Input: part model. Units: mm. Frame: model coordinates. A direction names the side the tool comes from. Round coordinates to 2 decimals unless told otherwise and drop trailing zeros. Order: outer loops, then holes, each group sorted by start corner. A loop starts at its lowest first (then second) coordinate and runs counter-clockwise, first axis right, second up. Notation, with made-up numbers: (70.5, -33) -> (104.5, -33) arc R23 ccw to (104.5, -16) -> close; hole circle Ø3 at (57.5, -4.75). An arc over 180 degrees is marked (long way). Use a Markdown table: item, result.
from build123d import *

# Parameters (mm, degrees)
F0_W      = 1000
F0_H      = 1000
F1_DEPTH  = 300
F2_W      = 900
F2_H      = 100
F3_DEPTH  = 1000.001
F4_W      = 100
F4_H      = 900
F5_DEPTH  = 1000.001
F6_W      = 300
F6_H      = 120
F7_DEPTH  = 150
F8_W      = 300
F8_H      = 120
F9_DEPTH  = 150
F10_W     = 120
F10_H     = 300
F11_DEPTH = 150
F12_W     = 120
F12_H     = 300
F13_DEPTH = 150
F14_R     = 5
F15_R     = 5
F16_W     = 680
F16_H     = 680
F17_DEPTH = 300.001
F18_W     = 10
F18_H     = 680
F19_DEPTH = 160.001
F20_DEPTH = 840.001
F21_SCALE = 0.1


with BuildPart() as f1:
    # F0 (on Front) → F1 (new body)
    with BuildSketch(Plane.XZ):
        with Locations((450.7653813809, 448.8989327101)):
            Rectangle(F0_W, F0_H)
    extrude(amount=F1_DEPTH)

    # F2 (on face) → F3 (cut, through all)
    with BuildSketch(Plane.XY.offset(948.8989327101)):
        with Locations((450.7653813809, -250)):
            Rectangle(F2_W, F2_H)
    extrude(amount=-F3_DEPTH, mode=Mode.SUBTRACT)

    # F4 (on face) → F5 (cut, through all)
    with BuildSketch(Plane(origin=(-49.2346186191, 0, 0), x_dir=(0, -1, 0), z_dir=(-1, 0, 0))):
        with Locations((250, 448.8989327101)):
            Rectangle(F4_W, F4_H)
    extrude(amount=-F5_DEPTH, mode=Mode.SUBTRACT)

    # F6 (on face) → F7 (cut)
    with BuildSketch(Plane(origin=(0, 0, -51.1010672899), x_dir=(1, 0, 0), z_dir=(0, 0, -1))):
        with Locations((100.7653813809, 110)):
            Rectangle(F6_W, F6_H)
    extrude(amount=-F7_DEPTH, mode=Mode.SUBTRACT)

    # F8 (on face) → F9 (cut)
    with BuildSketch(Plane(origin=(0, 0, -51.1010672899), x_dir=(1, 0, 0), z_dir=(0, 0, -1))):
        with Locations((800.7653813809, 110)):
            Rectangle(F8_W, F8_H)
    extrude(amount=-F9_DEPTH, mode=Mode.SUBTRACT)

    # F10 (on face) → F11 (cut)
    with BuildSketch(Plane.YZ.offset(950.7653813809)):
        with Locations((-110, 798.8989327101)):
            Rectangle(F10_W, F10_H)
    extrude(amount=-F11_DEPTH, mode=Mode.SUBTRACT)

    # F12 (on face) → F13 (cut)
    with BuildSketch(Plane(origin=(-49.2346186191, 0, 0), x_dir=(0, -1, 0), z_dir=(-1, 0, 0))):
        with Locations((110, 798.8989327101)):
            Rectangle(F12_W, F12_H)
    extrude(amount=-F13_DEPTH, mode=Mode.SUBTRACT)

    # F14
    f14_edges = [f1.edges().sort_by_distance(p)[0] for p in [
        (950.765381, -235, -51.101067),
        (900.765381, -250, -51.101067),
        (950.765381, -250, -1.101067),
        (900.765381, -250, -1.101067),
        (-49.234619, -235, -51.101067),
        (0.765381, -250, -51.101067),
        (-49.234619, -250, -1.101067),
        (0.765381, -250, -1.101067),
        (-49.234619, -235, 948.898933),
        (0.765381, -250, 948.898933),
        (-49.234619, -250, 898.898933),
        (0.765381, -250, 898.898933),
        (950.765381, -235, 948.898933),
        (950.765381, -250, 898.898933),
        (900.765381, -250, 898.898933),
        (900.765381, -250, 948.898933),
    ]]
    fillet(f14_edges, radius=F14_R)

    # F15
    f15_edges = [f1.edges().sort_by_distance(p)[0] for p in [
        (950.765381, -25, 948.898933),
        (950.765381, -25, -51.101067),
        (-49.234619, -25, -51.101067),
        (-49.234619, -25, 948.898933),
    ]]
    fillet(f15_edges, radius=F15_R)

    # F16 (on face) → F17 (cut, through all)
    with BuildSketch(Plane(origin=(0, 0, 0), x_dir=(-1, 0, 0), z_dir=(0, 1, 0))):
        with Locations((-450.7653813809, 448.8989327101)):
            Rectangle(F16_W, F16_H)
    extrude(amount=-F17_DEPTH, mode=Mode.SUBTRACT)

    # F18 (on face) → F19 (cut, through all)
    with BuildSketch(Plane.YZ.offset(110.7653813809)):
        with Locations((-10, 445.622831583)):
            Rectangle(F18_W, F18_H)
    extrude(amount=-F19_DEPTH, mode=Mode.SUBTRACT)

    # F18 (on face) → F20 (cut, through all)
    with BuildSketch(Plane.YZ.offset(110.7653813809)):
        with Locations((-10, 445.622831583)):
            Rectangle(F18_W, F18_H)
    extrude(amount=F20_DEPTH, mode=Mode.SUBTRACT)


with BuildPart() as f1_1:
    # F21: moved
    add(f1.part.scale(F21_SCALE))


solid = f1_1.part
1) Cut plane B-B on x = 13.5. Return loops of the section in (y, z), and give its area (3 significant figures).
Results found:
| item | result |
|---|---|
| outline | (-20, -5.11) -> (-17, -5.11) -> (-17, 9.89) -> (-5, 9.89) -> (-5, -5.11) -> (0, -5.11) -> (0, 10.89) -> (-0.5, 10.89) -> (-0.5, 10.56) -> (-1.5, 10.56) -> (-1.5, 10.89) -> (-20, 10.89) -> close; (-20, 78.89) -> (0, 78.89) -> (0, 94.89) -> (-20, 94.89) -> close |
| area | 460 mm² |
2) Cut plane A-A on y = -24.25. Count the separate pieces of the cut face and the enclosed holes in it, and give its area (3 significant figures).
Results found:
| item | result |
|---|---|
| separate pieces | 4 |
| enclosed holes | 0 |
| area | 99.1 mm² |
3) Set-up query: faces 1 (the flat face through (10, -5, 2)), 2 (the flat face through (-2, -25, -0.11)), 3 (the flat face through (11.077, -12, 44)). Return all of +Z, -Z, +X, -X, +Y, -Y with unobstructed straight access to the full face (end or side cutting, diameter ignored); none if empty.
Results found:
| item | result |
|---|---|
| face 1 | -Z, -X |
| face 2 | +X, -X, -Y |
| face 3 | +Y, -Y |
4) Pull-direction query (Y, two-part tool) for faces 4 (the flat face through (-4.923, -11, 44)), 5 (the flat face through (-2, -30, -3)), 6 (the flat face through (80, -11, 9.89)), 7 (the flat face through (8, -1.5, 42)); classes: +Y half, -Y half, draft (parallel to the pull), parting line (faces both ways), or undercut.
Results found:
| item | result |
|---|---|
| face 4 | draft |
| face 5 | -Y half |
| face 6 | undercut |
| face 7 | undercut |
5) Pin query (flat end, axial travel): pin 1 Ø6 at (x, y) = (76.5, -9.5) entering from -Z; pin 2 Ø12 at (x, z) = (10.5, 5.5) entering from -Y; pin 3 Ø3.5 at (x, y) = (90, -13.5) entering from +Z. Return the tip coordinate at first contact, or that it passes through.
Results found:
| item | result |
|---|---|
| pin 1 | stops at z = 9.89 |
| pin 2 | stops at y = -20 |
| pin 3 | stops at z = 64.89 |
6) Cut plane D-D on y = -11.25. Return loops of the section in (x, z).
Results found:
| item | result |
|---|---|
| outline | (-4.92, 9.89) -> (25.08, 9.89) -> (25.08, -5.11) -> (65.08, -5.11) -> (65.08, 9.89) -> (95.08, 9.89) -> (95.08, 64.89) -> (80.08, 64.89) -> (80.08, 94.89) -> (10.08, 94.89) -> (10.08, 64.89) -> (-4.92, 64.89) -> close; hole (11.08, 10.89) -> (79.08, 10.89) -> (79.08, 78.89) -> (11.08, 78.89) -> close |
7) Cut plane C-C on z = 33. Return loops of the section in (x, y).
Results found:
| item | result |
|---|---|
| outline | (-4.92, -20) -> (11.08, -20) -> (11.08, -1.5) -> (-4.92, -1.5) -> close; (-4.92, -0.5) -> (11.08, -0.5) -> (11.08, 0) -> (-4.92, 0) -> close; (79.08, -20) -> (95.08, -20) -> (95.08, -1.5) -> (79.08, -1.5) -> close; (79.08, -0.5) -> (95.08, -0.5) -> (95.08, 0) -> (79.08, 0) -> close |
8) Line query: L1, parallel to Y at x = 86, z = 7.5; L2, parallel to Z at x = 57.5, y = -13.5; L3, parallel to X at y = -5.75, z = 69. Output: solid intervals per line, ascending. Write a range as [from, to].
Results found:
| item | result |
|---|---|
| L1 | y = [-20, -17], [-5, 0] |
| L2 | z = [-5.11, 10.89], [78.89, 94.89] |
| L3 | x = [10.08, 11.08], [79.08, 80.08] |
